Part model, mm, in its own coordinate system. Face numbers are marked on the shaded views. Coordinates: 2 decimals unless noted, no trailing zeros. Write each loop counter-clockwise with the first axis right and the second up, starting at its lowest first coordinate (ties: lowest second). Pieces come first, ordered by that corner, then holes. Notation, with made-up numbers: M -19.75,27 L 33.25,27 A26 cw 33.25,52 Z; hole C 33,-12 d5. An arc over 180 degrees is marked long. Use a Markdown table: item, result. Add a question column.
Q1. Wall check: L1, parallel to X at y = -78, z = -1.1; L2, parallel to Y at x = 15, z = -0.55; L3, parallel to Y at x = 16, z = -1.5. Give the ranges that are in metal, low to high. Write a range as from..to.
Q2. Slice it at C-C on y = -6.5. Write the cut outline in (x, z).
Q3. Slice it at B-B on x = 15. Write the cut outline in (y, z), then the cut area to 3 significant figures.
Q4. Pin check, flat tips, straight feed: pin 1 Ø8 at (y, z) = (-10, -7.5) entering from +X; pin 2 Ø14.5 at (x, y) = (18.27, -12.73) entering from -Z; pin 3 Ø5.5 at (x, y) = (15, -36) entering from -Z. Stop position of each tip, or through.
Q5. Mould opens along X. For the marked faces 1, 2 and 3 say: released by +X, released by -X, zero draft, split by the parting line, or undercut.
Q6. Slice it at D-D on x = 25.25. Write the cut outline in (y, z).
Q7. Slice it at A-A on y = -78. Write the cut outline in (x, z), then the cut area to 3 significant figures.
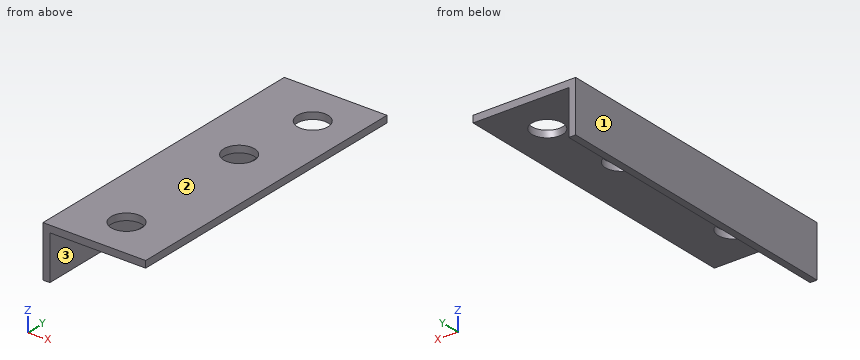
from build123d import *

# Parameters (mm, degrees)
F1_DEPTH = 90
F2_R     = 4.5
F3_DEPTH = 2.001
F4_R     = 4.5
F5_DEPTH = 15.001


with BuildPart() as f1:
    # F0 (on Front) → F1 (new body)
    with BuildSketch(Plane.XZ):
        Polygon((0, 0), (0, -15), (2, -15), (2, -2), (30, -2), (30, 0), align=None)
    extrude(amount=F1_DEPTH)

    # F2 (on face) → F3 (cut, through all)
    with BuildSketch(Plane(origin=(0, 0, -2), x_dir=(1, 0, 0), z_dir=(0, 0, -1))):
        with Locations((15, 78)):
            Circle(F2_R)
        with Locations((15, 36)):
            Circle(F2_R)
    extrude(amount=-F3_DEPTH, mode=Mode.SUBTRACT)

    # F4 (on face) → F5 (cut, through all)
    with BuildSketch(Plane.XY):
        with Locations((18.270568, -12.7287)):
            Circle(F4_R)
    extrude(amount=-F5_DEPTH, mode=Mode.SUBTRACT)


solid = f1.part
Recorded:
| question | item | result |
|---|---|---|
| 1 | L1 | 0..10.5, 19.5..30 |
| 1 | L2 | -90..-82.5, -73.5..-40.5, -31.5..-15.82, -9.64..0 |
| 1 | L3 | -90..-82.39, -73.61..-40.39, -31.61..-16.61, -8.84..0 |
| 2 | outline | M 0,-15 L 2,-15 L 2,-2 L 30,-2 L 30,0 L 0,0 Z |
| 3 | outline | M -90,-2 L -82.5,-2 L -82.5,0 L -90,0 Z; M -73.5,-2 L -40.5,-2 L -40.5,0 L -73.5,0 Z; M -31.5,-2 L -15.82,-2 L -15.82,0 L -31.5,0 Z; M -9.64,-2 L 0,-2 L 0,0 L -9.64,0 Z |
| 3 | area | 132 mm² |
| 4 | pin 1 | x = 2 |
| 4 | pin 2 | z = -2 |
| 4 | pin 3 | through |
| 5 | face 1 | released by -X |
| 5 | face 2 | zero draft |
| 5 | face 3 | released by +X |
| 6 | outline | M -90,-2 L 0,-2 L 0,0 L -90,0 Z |
| 7 | outline | M 0,-15 L 2,-15 L 2,-2 L 10.5,-2 L 10.5,0 L 0,0 Z; M 19.5,-2 L 30,-2 L 30,0 L 19.5,0 Z |
| 7 | area | 68.0 mm² |
